Job drawing, mm, ordinate dimensions from the low corner. One solid piece. Give positions to 0.01 mm unless a question says otherwise; leave off trailing zeros. Write each loop counter-clockwise with the first axis right and the second up, starting at its lowest first coordinate (ties: lowest second). Pieces come first, ordered by that corner, then holes. Notation, with made-up numbers: (55, 44.5) - (74, 44.5) arc R18 cw to (74, 62.5) - close; hole circle Ø7 at (77.25, -26). An arc over 180 degrees is marked (long way). Answer as a JSON object with one key per item and string values.
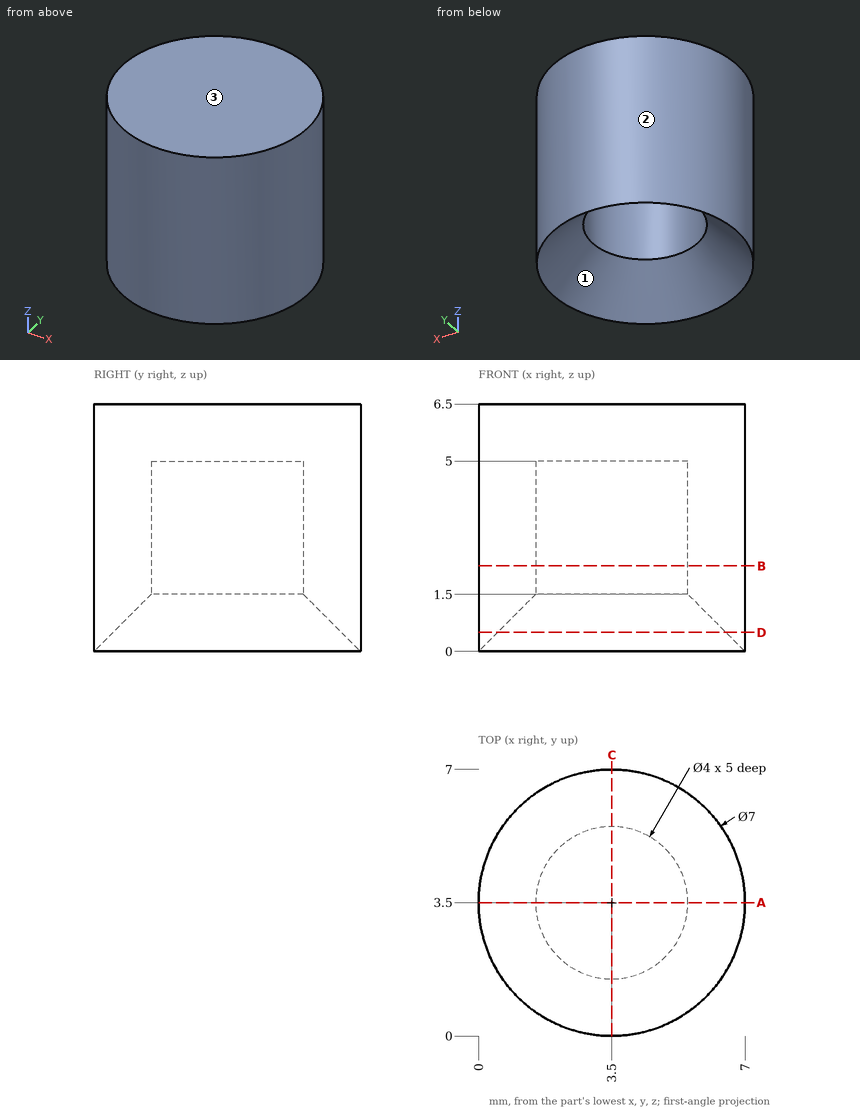
Item 1: Probe line 1 (Y direction, x = 3.5, z = 3.45); line 2 (Y direction, x = 5, z = 3.75); line 3 (X direction, y = 4, z = 2.5). List the from-to ranges inside material, lowest first. Write a range as from..to.
Entries:
{"line 1": "0..1.5, 5.5..7", "line 2": "0.34..2.18, 4.82..6.66", "line 3": "0.04..1.56, 5.44..6.96"}
Item 2: Cut at A-A (y = 3.5). Give the cut face in (x, z).
Entries:
{"outline": "(0, 0) - (1.5, 1.5) - (1.5, 5) - (5.5, 5) - (5.5, 1.5) - (7, 0) - (7, 6.5) - (0, 6.5) - close"}
Item 3: Cut at B-B (z = 2.25). Give the cut face in (x, y).
Entries:
{"outline": "circle Ø7 at (3.5, 3.5); hole circle Ø4 at (3.5, 3.5)"}
Item 4: Cut at D-D (z = 0.5). Give the cut face in (x, y).
Entries:
{"outline": "circle Ø7 at (3.5, 3.5); hole circle Ø6 at (3.5, 3.5)"}
Item 5: Flat gauge pin, fed straight in: P1, Ø2, axis at x = 3.5, y = 3, coming from the -Z side. Where does the tip first touch, or does it go through?
Entries:
{"P1": "z = 5"}
Item 6: Mould opens along X. For the marked faces 1, 2 and 3 say: +X half, -X half, draft (parallel to the pull), parting line (faces both ways), or undercut.
Entries:
{"face 1": "undercut", "face 2": "parting line", "face 3": "draft"}
